```python
from build123d import *

# Parameters (mm, degrees)
SKETCH_1_W                       = 400
SKETCH_1_H                       = 610
EXTRUDE_1_DEPTH                  = 16
SKETCH_2_R                       = 13
CUT_EXTRUDE_1_DEPTH              = 730.627302121
PATTERN_LINEAR_1_COUNT           = 2
PATTERN_LINEAR_1_PITCH           = 300
PATTERN_LINEAR_1_COUNT_DIR2      = 6
PATTERN_LINEAR_1_PITCH_DIR2      = 80
SKETCH_3_W                       = 16
SKETCH_3_H                       = 650
EXTRUDE_2_DEPTH                  = 216
SKETCH_4_R                       = 13
CUT_EXTRUDE_2_DEPTH              = 721.824527885
SKETCH_5_W                       = 400
SKETCH_5_H                       = 10
EXTRUDE_3_DEPTH                  = 216
CUT_EXTRUDE_3_DEPTH              = 619
SKETCH_7_W                       = 400
SKETCH_7_H                       = 10
EXTRUDE_4_DEPTH                  = 132
CUT_EXTRUDE_4_DEPTH              = 10
SKETCH_9_W                       = 298
SKETCH_9_H                       = 240
EXTRUDE_5_DEPTH                  = 16
SKETCH_10_R                      = 13
CUT_EXTRUDE_5_DEPTH              = 16
PATTERN_LINEAR_2_COUNT           = 2
PATTERN_LINEAR_2_PITCH           = 80
PATTERN_LINEAR_3_COUNT           = 2
PATTERN_LINEAR_3_PITCH           = 200
PATTERN_LINEAR_4_COUNT           = 3
PATTERN_LINEAR_4_PITCH           = 80
PATTERN_LINEAR_4_COPY_1_SKETCH_R = 13
PATTERN_LINEAR_4_COPY_1_DEPTH    = 16
PATTERN_LINEAR_4_COPY_2_SKETCH_R = 13
PATTERN_LINEAR_4_COPY_2_DEPTH    = 16
PATTERN_LINEAR_4_COPY_3_SKETCH_R = 13
PATTERN_LINEAR_4_COPY_3_DEPTH    = 16
PATTERN_LINEAR_4_COPY_4_SKETCH_R = 13
PATTERN_LINEAR_4_COPY_4_DEPTH    = 16
EXTRUDE_START                    = 11.5
SKETCH_12_W                      = 90
SKETCH_12_H                      = 240
SKETCH_12_R                      = 13
EXTRUDE_6_DEPTH                  = 11.5
SKETCH_11_W                      = 259.5
SKETCH_11_H                      = 650
CUT_EXTRUDE_6_DEPTH              = 807.126695998


with BuildPart() as part:
    # 草图1 → 凸台-拉伸1 (new body)
    with BuildSketch(Plane.XY):
        with Locations((200, 305)):
            Rectangle(SKETCH_1_W, SKETCH_1_H)
    extrude(amount=EXTRUDE_1_DEPTH)

    # 草图2 → 切除-拉伸1 (cut, through all)
    with BuildSketch(Plane.XY.offset(16)):
        with Locations((50, 50)):
            Circle(SKETCH_2_R)
    cut_extrude_1 = extrude(amount=-CUT_EXTRUDE_1_DEPTH, mode=Mode.SUBTRACT)

    # 阵列(线性)1: Cut-Extrude 1 2 × 6
    with Locations(*[(i * PATTERN_LINEAR_1_PITCH, j * PATTERN_LINEAR_1_PITCH_DIR2, 0) for i in range(PATTERN_LINEAR_1_COUNT) for j in range(PATTERN_LINEAR_1_COUNT_DIR2) if (i, j) != (0, 0)]):
        add(cut_extrude_1, mode=Mode.SUBTRACT)

    # 草图3 → 凸台-拉伸2 (add)
    with BuildSketch(Plane.XY.offset(16)):
        with Locations((200, 325)):
            Rectangle(SKETCH_3_W, SKETCH_3_H)
    extrude(amount=EXTRUDE_2_DEPTH)

    # 草图4 → 切除-拉伸2 (cut, through all)
    with BuildSketch(Plane(origin=(208, 0, 0), x_dir=(0, 0, -1), z_dir=(1, 0, 0))):
        with Locations((-93.5, 210)):
            Circle(SKETCH_4_R)
        with Locations((-93.5, 130)):
            Circle(SKETCH_4_R)
        with Locations((-93.5, 50)):
            Circle(SKETCH_4_R)
        Polygon((-232, 650), (-16, 650), (-16, 610), align=None)
        with BuildLine():
            Line((-198.5, 410), (-232, 410))
            Line((-232, 410), (-232, 0))
            Line((-232, 0), (-148.5, 0))
            Line((-148.5, 0), (-148.5, 360))
            ThreePointArc((-148.5, 360), (-163.144660941, 395.355339059), (-198.5, 410))
        make_face()
    extrude(amount=-CUT_EXTRUDE_2_DEPTH, mode=Mode.SUBTRACT)

    # 草图5 → 凸台-拉伸3 (add)
    with BuildSketch(Plane.XY.offset(16)):
        with Locations((200, 570)):
            Rectangle(SKETCH_5_W, SKETCH_5_H)
        with Locations((200, 490)):
            Rectangle(SKETCH_5_W, SKETCH_5_H)
        with Locations((200, 415)):
            Rectangle(SKETCH_5_W, SKETCH_5_H)
    extrude(amount=EXTRUDE_3_DEPTH)

    # 草图6 → 切除-拉伸3 (cut, through all)
    with BuildSketch(Plane(origin=(0, 410, 0), x_dir=(-1, 0, 0), z_dir=(0, -1, 0))):
        with BuildLine():
            Line((-298, -232), (-298, -114.300395022))
            ThreePointArc((-298, -114.300395022), (-306.001372744, -87.168950007), (-327.444612345, -68.721057178))
            Line((-327.444612345, -68.721057178), (-400, -36))
            Line((-400, -36), (-400, -232))
            Line((-400, -232), (-298, -232))
        make_face()
    extrude(amount=-CUT_EXTRUDE_3_DEPTH, mode=Mode.SUBTRACT)

    # 草图7 → 凸台-拉伸4 (add)
    with BuildSketch(Plane.XY.offset(16)):
        with Locations((200, 330)):
            Rectangle(SKETCH_7_W, SKETCH_7_H)
    extrude(amount=EXTRUDE_4_DEPTH)

    # 草图8 → 切除-拉伸4 (cut)
    with BuildSketch(Plane(origin=(0, 325, 0), x_dir=(-1, 0, 0), z_dir=(0, -1, 0))):
        Polygon((-400, -148), (-300, -148), (-400, -76), align=None)
        Polygon((0, -148), (-100, -148), (0, -76), align=None)
    extrude(amount=-CUT_EXTRUDE_4_DEPTH, mode=Mode.SUBTRACT)

    # 草图9 → 凸台-拉伸5 (add)
    with BuildSketch(Plane.XY.offset(232)):
        with Locations((149, 530)):
            Rectangle(SKETCH_9_W, SKETCH_9_H)
    extrude(amount=EXTRUDE_5_DEPTH)

    # 草图10 → 切除-拉伸5 (cut)
    with BuildSketch(Plane.XY.offset(248)):
        with Locations((60, 610)):
            Circle(SKETCH_10_R)
    cut_extrude_5 = extrude(amount=-CUT_EXTRUDE_5_DEPTH, mode=Mode.SUBTRACT)

    # 阵列(线性)2: 切除-拉伸5 ×2
    with Locations(*[(i * PATTERN_LINEAR_2_PITCH, 0, 0) for i in range(1, PATTERN_LINEAR_2_COUNT)]):
        add(cut_extrude_5, mode=Mode.SUBTRACT)

    # 阵列(线性)3: 切除-拉伸5 ×2
    with Locations(*[(i * PATTERN_LINEAR_3_PITCH, 0, 0) for i in range(1, PATTERN_LINEAR_3_COUNT)]):
        add(cut_extrude_5, mode=Mode.SUBTRACT)

    # 阵列(线性)4: 切除-拉伸5 ×3
    with Locations(*[(0, -i * PATTERN_LINEAR_4_PITCH, 0) for i in range(1, PATTERN_LINEAR_4_COUNT)]):
        add(cut_extrude_5, mode=Mode.SUBTRACT)

    # 阵列(线性)4 copy 1 sketch → 阵列(线性)4 copy 1 (cut)
    with BuildSketch(Plane(origin=(80, -80, 248), x_dir=(1, 0, 0), z_dir=(0, 0, 1))):
        with Locations((60, 610)):
            Circle(PATTERN_LINEAR_4_COPY_1_SKETCH_R)
    extrude(amount=-PATTERN_LINEAR_4_COPY_1_DEPTH, mode=Mode.SUBTRACT)

    # 阵列(线性)4 copy 2 sketch → 阵列(线性)4 copy 2 (cut)
    with BuildSketch(Plane(origin=(80, -160, 248), x_dir=(1, 0, 0), z_dir=(0, 0, 1))):
        with Locations((60, 610)):
            Circle(PATTERN_LINEAR_4_COPY_2_SKETCH_R)
    extrude(amount=-PATTERN_LINEAR_4_COPY_2_DEPTH, mode=Mode.SUBTRACT)

    # 阵列(线性)4 copy 3 sketch → 阵列(线性)4 copy 3 (cut)
    with BuildSketch(Plane(origin=(200, -80, 248), x_dir=(1, 0, 0), z_dir=(0, 0, 1))):
        with Locations((60, 610)):
            Circle(PATTERN_LINEAR_4_COPY_3_SKETCH_R)
    extrude(amount=-PATTERN_LINEAR_4_COPY_3_DEPTH, mode=Mode.SUBTRACT)

    # 阵列(线性)4 copy 4 sketch → 阵列(线性)4 copy 4 (cut)
    with BuildSketch(Plane(origin=(200, -160, 248), x_dir=(1, 0, 0), z_dir=(0, 0, 1))):
        with Locations((60, 610)):
            Circle(PATTERN_LINEAR_4_COPY_4_SKETCH_R)
    extrude(amount=-PATTERN_LINEAR_4_COPY_4_DEPTH, mode=Mode.SUBTRACT)

    # 草图12 → 凸台-拉伸6 (add)
    with BuildSketch(Plane.XY.offset(248).offset(EXTRUDE_START)):
        with Locations((253, 530)):
            Rectangle(SKETCH_12_W, SKETCH_12_H)
        with Locations((260, 610)):
            Circle(SKETCH_12_R, mode=Mode.SUBTRACT)
        with Locations((260, 530)):
            Circle(SKETCH_12_R, mode=Mode.SUBTRACT)
        with Locations((260, 450)):
            Circle(SKETCH_12_R, mode=Mode.SUBTRACT)
    extrude(amount=-EXTRUDE_6_DEPTH)

    # 镜向1: part across plane


with BuildPart() as part_1:
    add(part.part)
    add(part.part.mirror(Plane.XY))

    # 草图11 → 切除-拉伸6 (cut, through all)
    with BuildSketch(Plane.ZY):
        with Locations((129.75, 325)):
            Rectangle(SKETCH_11_W, SKETCH_11_H)
    extrude(amount=-CUT_EXTRUDE_6_DEPTH, mode=Mode.SUBTRACT)


solid = part_1.part
```
The model under review builds one solid part; all positions refer to its coordinate system, in mm. A direction names the side the tool comes from. Round coordinates to 2 decimals unless told otherwise and drop trailing zeros. Order: outer loops, then holes, each group sorted by start corner. A loop starts at its lowest first (then second) coordinate and runs counter-clockwise, first axis right, second up.
(1) Take a section at C-C, the plane y = 450. Count the separate pieces of the cut face and the enclosed holes in it, plus the area to 3 significant figures.
Working result:
separate pieces: 6
enclosed holes: 0
area: 13,300 mm2
(2) For P1, Ø4, axis at y = 548, z = -48.5, coming from the +X side; P2, Ø5, axis at x = 78, z = -50.5, coming from the +Y side; P3, Ø10, axis at y = 547.5, z = -162, coming from the -X side; P4, Ø15.5, axis at x = 350, y = 210, coming from the -Z side, all flat-tipped, find the tip position at first contact; note any pin that passes through.
Working result:
P1: stops at x = 208
P2: stops at y = 575
P3: stops at x = 192
P4: passes through
(3) Take a section at B-B, the plane y = 530. State the section outline as (x, z) points, plus the area to 3 significant figures.
Working result:
outline: (0, -248) - (47, -248) - (47, -232) - (0, -232) - close; (0, -16) - (192, -16) - (192, -232) - (153, -232) - (153, -248) - (208, -248) - (208, -259.5) - (247, -259.5) - (247, -232) - (208, -232) - (208, -16) - (400, -16) - (400, 0) - (0, 0) - close; (73, -248) - (127, -248) - (127, -232) - (73, -232) - close; (273, -259.5) - (298, -259.5) - (298, -232) - (273, -232) - close
area: 14,100 mm2
(4) Tool access review of faces 4 (the face through (95, 575, -122)), 5 (the face through (197, 610, -8)), 6 (the face through (303, 325, -81)), 7 (the face through (303, 593, -16)), 8 (the face through (192, 452, -122)): name each direction out of +Z, -Z, +X, -X, +Y, -Y from which nothing blocks a thin tool from reaching the whole face with its end or side.
Working result:
face 4: -X, +Y
face 5: +Z, +X, -X, +Y
face 6: -Z, +X, -Y
face 7: +X, +Y
face 8: -X
(5) Mouldability with a two-part tool opening along Z and no side actions: class faces 1 (the face through (305.785, 414.93, -87.507)), 2 (the face through (95, 485, -122)), 3 (the face through (347.18, 117.31, -8.11)) as released by +Z, released by -Z, zero draft, split by the parting line, or undercut.
Working result:
face 1: released by -Z
face 2: undercut
face 3: zero draft
(6) Take a section at D-D, the plane z = -169.5. State the section outline as (x, y) points, plus the area to 3 significant figures.
Working result:
outline: (0, 410) - (192, 410) - (192, 400.73) - (208, 400.73) - (208, 410) - (298, 410) - (298, 420) - (208, 420) - (208, 485) - (298, 485) - (298, 495) - (208, 495) - (208, 565) - (298, 565) - (298, 575) - (208, 575) - (208, 638.43) - (192, 638.43) - (192, 575) - (0, 575) - (0, 565) - (192, 565) - (192, 495) - (0, 495) - (0, 485) - (192, 485) - (192, 420) - (0, 420) - close
area: 12,300 mm2
(7) Wall thickness on L1, parallel to X at y = 210, z = -11; L2, parallel to X at y = 610, z = -237; L3, parallel to Y at x = 290.5, z = -130: over which ranges is each line inside the solid? List them lowest first.
Working result:
L1: x = 0 to 37, 63 to 337, 363 to 400
L2: x = 0 to 47, 73 to 127, 153 to 247, 273 to 298
L3: y = 325 to 335, 410 to 420, 485 to 495, 565 to 575
